Verification items for this drawing (mm, ordinates from the low corner). Round coordinates to 2 decimals unless told otherwise and drop trailing zeros. Write each loop counter-clockwise with the first axis right and the second up, starting at its lowest first coordinate (ties: lowest second). Pieces come first, ordered by that corner, then holes. Notation, with made-up numbers: (45, 85) -> (99, 85) arc R16 ccw to (99, 101) -> close; hole circle Ø8 at (-30.5, 71.25). An arc over 180 degrees is marked (long way). Return JSON: item names as keys, results as strings. Group by question number.
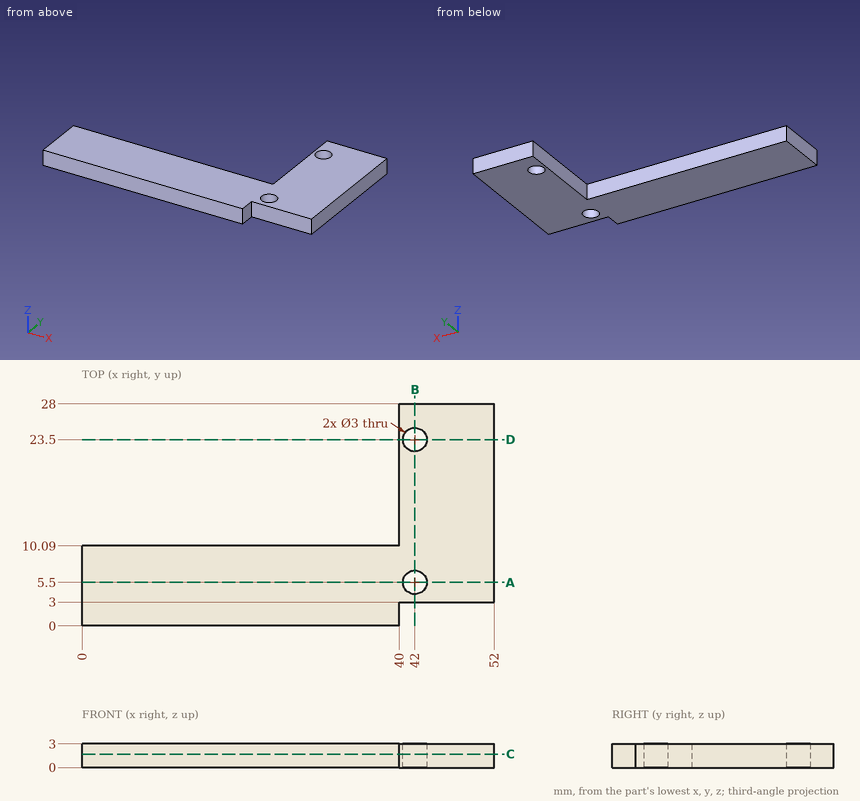
1) Sectioned sample at A-A on y = 5.5. Enter the section's corners in (x, z).
2) Sectioned sample at C-C on z = 1.7. Enter the section's corners in (x, y).
3) Sectioned sample at D-D on y = 23.5. Enter the section's corners in (x, z), and give its area (3 significant figures).
4) Material ranges on probe 1 along Y at (x, z) = (42, 2.3); probe 2 along Y at (x, z) = (42.5, 0.3) (1 decimal); probe 3 along X at (y, z) = (11.25, 2.8), recorded low to high. Write a range as [from, to].
5) Sectioned sample at B-B on x = 42. Enter the section's corners in (y, z), and give its area (3 significant figures).
6) Go/stop test with flat-tipped pins: P1, Ø0.9, axis at x = 15.5, z = 2, coming from the +Y side; P2, Ø2.5, axis at x = 42, y = 23.5, coming from the +Z side; P3, Ø1.5, axis at y = 12, z = 1, coming from the -X side; P4, Ø0.9, axis at y = 1.5, z = 2, coming from the +X side. Record where each tip stops, or that it passes through.
Evaluation:
{
 "1": {"outline": "(0, 0) -> (40.5, 0) -> (40.5, 3) -> (0, 3) -> close; (43.5, 0) -> (52, 0) -> (52, 3) -> (43.5, 3) -> close"},
 "2": {"outline": "(0, 0) -> (40, 0) -> (40, 3) -> (52, 3) -> (52, 28) -> (40, 28) -> (40, 10.09) -> (0, 10.09) -> close; hole circle Ø3 at (42, 5.5); hole circle Ø3 at (42, 23.5)"},
 "3": {"outline": "(40, 0) -> (40.5, 0) -> (40.5, 3) -> (40, 3) -> close; (43.5, 0) -> (52, 0) -> (52, 3) -> (43.5, 3) -> close", "area": "27.0 mm2"},
 "4": {"probe 1": "y = [3, 4], [7, 22], [25, 28]", "probe 2": "y = [3, 4.1], [6.9, 22.1], [24.9, 28]", "probe 3": "x = [40, 52]"},
 "5": {"outline": "(3, 0) -> (4, 0) -> (4, 3) -> (3, 3) -> close; (7, 0) -> (22, 0) -> (22, 3) -> (7, 3) -> close; (25, 0) -> (28, 0) -> (28, 3) -> (25, 3) -> close", "area": "57.0 mm2"},
 "6": {"P1": "stops at y = 10.09", "P2": "passes through", "P3": "stops at x = 40", "P4": "stops at x = 40"}
}
